Part model, mm, in its own coordinate system. Face numbers are marked on the shaded views. A direction names the side the tool comes from. Round coordinates to 2 decimals unless told otherwise and drop trailing zeros. Order: outer loops, then holes, each group sorted by start corner. A loop starts at its lowest first (then second) coordinate and runs counter-clockwise, first axis right, second up. Notation, with made-up numbers: (47.25, 83.5) - (97.25, 83.5) arc R14 cw to (97.25, 105.5) - close; hole circle Ø3 at (-18, 22.5). An arc over 180 degrees is marked (long way). Return JSON: item names as keys, results as strings. Group by question number.
Item 1: Probe probe 1 along Z at (x, y) = (14.25, 2.25); probe 2 along Y at (x, z) = (15, 3); probe 3 along Y at (x, z) = (5, 15). List the from-to ranges inside material, lowest first.
Item 2: Tool access for the marked faces 4, 5 and 6: list every direction of +Z, -Z, +X, -X, +Y, -Y with a clear straight run to the whole face (end or side of a thin tool).
Item 3: Two-plate mould, pull along Z, no slides. Class the marked faces 1, 2 and 3: released by +Z, released by -Z, zero draft, split by the parting line, or undercut.
Item 4: Drop flat-ended pins along their axis: pin 1 (1 mm diameter, centred on x = 6, y = 2.5, fed in from -Z); pin 2 (0.9 mm diameter, centred on x = 10.5, z = -16.5, fed in from -Y); pin 3 (2 mm diameter, centred on x = 5.5, y = 3, fed in from +Z); pin 4 (5 mm diameter, centred on x = 4.5, z = -12, fed in from +Y). Give the stop position or say it passes through.
Item 5: Saw through at C-C on z = -2.5. List the corners of the cut face in (x, y).
Item 6: Saw through at D-D on y = 0.5. List the corners of the cut face in (x, z), and give its area (3 significant figures).
Item 7: Saw through at B-B on x = 2.75. List the corners of the cut face in (y, z), and give its area (3 significant figures).
Item 8: Saw through at A-A on y = 2. List the corners of the cut face in (x, z).
```python
from build123d import *

# Parameters (mm, degrees)
EXTRUDE_1_DEPTH = 20
FILLET_1_R      = 1
CHAMFER_1_SIZE  = 1


with BuildPart() as part:
    # 草图1 → 凸台-拉伸1 (new body)
    with BuildSketch(Plane(origin=(0, 0, 0), x_dir=(0, 0, -1), z_dir=(1, 0, 0))):
        Polygon((0, 0), (-12.5, 0), (-12.5, 6), (-17.5, 6), (-17.5, 5), (-13.5, 5), (-13.5, -1), (0, -1), (13.5, -1), (13.5, 5), (17.5, 5), (17.5, 6), (12.5, 6), (12.5, 0), align=None)
    extrude(amount=EXTRUDE_1_DEPTH)

    # 圆角1
    fillet_1_edges = [part.edges().sort_by_distance(p)[0] for p in [
        (10, -1, -13.5),
        (10, -1, 13.5),
        (10, 5, 13.5),
        (10, 6, 12.5),
        (10, 0, 12.5),
        (10, 0, -12.5),
        (10, 6, -12.5),
        (10, 5, -13.5),
    ]]
    fillet(fillet_1_edges, radius=FILLET_1_R)

    # 倒角1
    chamfer_1_edges = [part.edges().sort_by_distance(p)[0] for p in [
        (0, 5.5, 17.5),
        (0, 5.5, -17.5),
    ]]
    chamfer(chamfer_1_edges, length=CHAMFER_1_SIZE)


solid = part.part
```
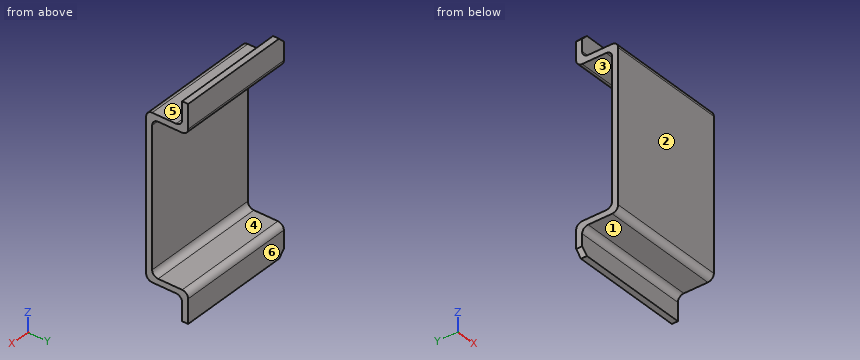
Filled in:
{
 "1": {"probe 1": "z = -13.5 to -12.5, 12.5 to 13.5", "probe 2": "y = -1 to 0", "probe 3": "y = 5 to 6"},
 "2": {"face 4": "+X, -X, +Y", "face 5": "+Z, +X, -X, -Y", "face 6": "+Z, -Z, +X, -X, +Y"},
 "3": {"face 1": "released by -Z", "face 2": "zero draft", "face 3": "undercut"},
 "4": {"pin 1": "stops at z = -13.5", "pin 2": "stops at y = 5", "pin 3": "stops at z = 13.5", "pin 4": "stops at y = 6"},
 "5": {"outline": "(0, -1) - (20, -1) - (20, 0) - (0, 0) - close"},
 "6": {"outline": "(0, -13.5) - (20, -13.5) - (20, -12.37) - (0, -12.37) - close; (0, 12.37) - (20, 12.37) - (20, 13.5) - (0, 13.5) - close", "area": "45.4 mm^2"},
 "7": {"outline": "(-1, -12.5) arc R1 ccw to (0, -13.5) - (4, -13.5) arc R1 cw to (5, -14.5) - (5, -17.5) - (6, -17.5) - (6, -13.5) arc R1 ccw to (5, -12.5) - (1, -12.5) arc R1 cw to (0, -11.5) - (0, 11.5) arc R1 cw to (1, 12.5) - (5, 12.5) arc R1 ccw to (6, 13.5) - (6, 17.5) - (5, 17.5) - (5, 14.5) arc R1 cw to (4, 13.5) - (0, 13.5) arc R1 ccw to (-1, 12.5) - close", "area": "47.0 mm^2"},
 "8": {"outline": "(0, -13.5) - (20, -13.5) - (20, -12.5) - (0, -12.5) - close; (0, 12.5) - (20, 12.5) - (20, 13.5) - (0, 13.5) - close"}
}
